Verification items for the finished model (mm, model axes). A direction names the side the tool comes from. Round coordinates to 2 decimals unless told otherwise and drop trailing zeros. Write each loop counter-clockwise with the first axis right and the second up, starting at its lowest first coordinate (ties: lowest second). Pieces come first, ordered by that corner, then holes. Notation, with made-up numbers: (85.5, 79) - (115.5, 79) arc R13 ccw to (115.5, 84) - close; hole circle Ø11 at (8, 24.5). An arc over 180 degrees is marked (long way). Answer as a JSON object with one key per item and string values.
```python
from build123d import *

# Parameters (mm, degrees)
SKETCH1_R           = 4.25
BOSS_EXTRUDE1_DEPTH = 114


with BuildPart() as part:
    # Sketch1 → Boss-Extrude1 (new body)
    with BuildSketch(Plane(origin=(0, 0, 0), x_dir=(1, 0, 0), z_dir=(0, 1, 0))):
        with Locations(Location((0, 0, 0), (0, 0, 90))):
            Circle(SKETCH1_R)
    extrude(amount=BOSS_EXTRUDE1_DEPTH)

    # Sketch2 → Revolve1 (revolve)
    with BuildSketch(Plane.XY, mode=Mode.PRIVATE) as revolve1_sk:
        with BuildLine():
            Line((2.25, 0), (2.25, -2))
            ThreePointArc((2.25, -2), (1.590990258, -3.590990258), (0, -4.25))
            Line((0, -4.25), (0, 0))
            Line((0, 0), (2.25, 0))
        make_face()
    revolve(revolve1_sk.sketch.rotate(Axis((0, 0, 0), (0, -1, 0)), 180), axis=Axis((0, 0, 0), (0, -1, 0)))

    # Sketch3 → Revolve2 (revolve)
    with BuildSketch(Plane.XY, mode=Mode.PRIVATE) as revolve2_sk:
        Polygon((0, 114), (0, 130), (4.25, 114), align=None)
    revolve(revolve2_sk.sketch.rotate(Axis((0, 114, 0), (0, 1, 0)), 90), axis=Axis((0, 114, 0), (0, 1, 0)))


solid = part.part
```
1. Access from +Z, -Z, +X, -X, +Y, -Y to the whole of each face (thin tool, end or side, straight path). Record for faces 3 (the face through (1.31, 121.89, 1.71)), 4 (the face through (1.66, -1.01, -1.52)).
Completed:
{"face 3": "+Y", "face 4": "-Y"}
2. Go/stop test with flat-tipped pins: pin 1 (1.5 mm diameter, centred on x = -2.5, y = 28, fed in from +Z); pin 2 (1.5 mm diameter, centred on x = -1.5, y = 69.5, fed in from +Z); pin 3 (5 mm diameter, centred on y = 56.5, z = 3, fed in from -X). Record where each tip stops, or that it passes through.
Completed:
{"pin 1": "stops at z = 3.87", "pin 2": "stops at z = 4.18", "pin 3": "stops at x = -4.22"}
3. Mould release check, pull along Z, two halves, no side actions. Record for faces 1 (the face through (-4.214, 56.202, 0.553)), 2 (the face through (2, 0, -2)): released by +Z, released by -Z, zero draft, split by the parting line, or undercut.
Completed:
{"face 1": "split by the parting line", "face 2": "zero draft"}
4. Cross-section at A-A (y = 94). Record the boundary of the cut face in (x, z).
Completed:
{"outline": "circle Ø8.5 at (0, 0)"}
5. Material ranges on probe 1 along Z at (x, y) = (-0.25, 110.5); probe 2 along X at (y, z) = (40.5, -1); probe 3 along Z at (x, y) = (3.5, 58), recorded low to high. Write a range as from..to.
Completed:
{"probe 1": "z = -4.24..4.24", "probe 2": "x = -4.13..4.13", "probe 3": "z = -2.41..2.41"}
